from build123d import *

# Parameters (mm, degrees)
SKETCH_1_R         = 30
SKETCH_1_R_2       = 8.75
EXTRUDE_1_DEPTH    = 4
HOLE_WIZARD_M6_1_D = 5


with BuildPart() as part:
    # 草图1 → 凸台-拉伸1 (new body)
    with BuildSketch(Plane.XY):
        Circle(SKETCH_1_R)
        Circle(SKETCH_1_R_2, mode=Mode.SUBTRACT)
    extrude(amount=EXTRUDE_1_DEPTH)

    # 草图4 → 旋转1 (revolve)
    with BuildSketch(Plane(origin=(0, 0, 0), x_dir=(1, 0, 0), z_dir=(0, 1, 0)), mode=Mode.PRIVATE) as revolve_1_sk:
        Polygon((-30, 0), (-30, 0.5), (-20, 0.5), (-18, 0), align=None)
    revolve(revolve_1_sk.sketch.rotate(Axis((0, 0, 0), (0, 0, -1)), 180), axis=Axis((0, 0, 0), (0, 0, -1)))

    # M6 螺纹孔1 (through all)
    with Locations(Plane.XY.offset(4)):
        with Locations((0, 15), (15, 0), (0, -15), (-15, 0)):
            Hole(HOLE_WIZARD_M6_1_D / 2)


solid = part.part
Model file for the job. Use its own axes, mm. A direction names the side the tool comes from. Give positions to 0.01 mm unless a question says otherwise; leave off trailing zeros. Loops run counter-clockwise (first coordinate to the right, second up) from the corner with the lowest first, then second, coordinate; pieces in that order, holes last. Notation, with made-up numbers: (60.25, 86) -> (76.25, 86) arc R13 ccw to (76.25, 103) -> close; hole circle Ø10 at (-30.5, 15.25). An arc over 180 degrees is marked (long way). Use a Markdown table: item, result. Add a question column.
(1) Drop flat-ended pins along their axis: pin 1 Ø2 at (x, z) = (1.5, 0) entering from -Y; pin 2 Ø8 at (x, y) = (15, 0) entering from -Z; pin 3 Ø1.5 at (x, z) = (9, 3.5) entering from -Y. Give the stop position or say it passes through.
(2) Slice it at C-C on y = -22.5. List the corners of the cut face in (x, z).
(3) Mould opens along Y. For faces 1 (the cylindrical face through (16.128, -25.296, 1.719)), 2 (the cylindrical face through (0.54, 12.56, 1.97)), 3 (the flat face through (6, 20, -0.5)) say: +Y half, -Y half, draft (parallel to the pull), parting line (faces both ways), or undercut.
(4) Slice it at D-D on x = -22. List the corners of the cut face in (y, z), and give its area (3 significant figures).
(5) Wall check: line 1 along Y through (x, z) = (0, 1.2); line 2 along Y through (x, z) = (0.5, 0.8). Give the ranges that are in metal, low to high.
(6) Tool access for faces 4 (the flat face through (-4, -8, 0)), 5 (the cylindrical face through (-12.5, 0.1, 2)): list every direction of +Z, -Z, +X, -X, +Y, -Y with a clear straight run to the whole face (end or side of a thin tool).
(7) Slice it at B-B on z = 2.5. List the corners of the cut face in (x, y).
(8) Slice it at A-A on y = 0. List the corners of the cut face in (x, z).
Filled sheet:
| question | item | result |
|---|---|---|
| 1 | pin 1 | y = -30 |
| 1 | pin 2 | z = -0.25 |
| 1 | pin 3 | y = -28.84 |
| 2 | outline | (-19.84, -0.5) -> (19.84, -0.5) -> (19.84, 4) -> (-19.84, 4) -> close |
| 3 | face 1 | parting line |
| 3 | face 2 | undercut |
| 3 | face 3 | draft |
| 4 | outline | (-20.4, -0.5) -> (20.4, -0.5) -> (20.4, 4) -> (-20.4, 4) -> close |
| 4 | area | 184 mm2 |
| 5 | line 1 | -30 to -17.5, -12.5 to -8.75, 8.75 to 12.5, 17.5 to 30 |
| 5 | line 2 | -30 to -17.45, -12.55 to -8.74, 8.74 to 12.55, 17.45 to 30 |
| 6 | face 4 | -Z |
| 6 | face 5 | +Z, -Z |
| 7 | outline | circle Ø60 at (0, 0); hole circle Ø5 at (-15, 0); hole circle Ø17.5 at (0, 0); hole circle Ø5 at (0, -15); hole circle Ø5 at (0, 15); hole circle Ø5 at (15, 0) |
| 8 | outline | (-30, -0.5) -> (-20, -0.5) -> (-18, 0) -> (-17.5, 0) -> (-17.5, 4) -> (-30, 4) -> close; (-12.5, 0) -> (-8.75, 0) -> (-8.75, 4) -> (-12.5, 4) -> close; (8.75, 0) -> (12.5, 0) -> (12.5, 4) -> (8.75, 4) -> close; (17.5, 0) -> (18, 0) -> (20, -0.5) -> (30, -0.5) -> (30, 4) -> (17.5, 4) -> close |
